from build123d import *

# Parameters (mm, degrees)
SKETCH1_R           = 3.95
BOSS_EXTRUDE1_DEPTH = 7.62
BOSS_EXTRUDE2_DEPTH = 7.62
BOSS_EXTRUDE3_DEPTH = 7.62
CUT_EXTRUDE1_DEPTH  = 7.62
SKETCH6_R           = 1.27
CUT_EXTRUDE2_DEPTH  = 4.9500048
SKETCH7_R           = 4.445
BOSS_EXTRUDE4_DEPTH = 1.27
FILLET1_R           = 2.54


with BuildPart() as part:
    # Sketch1 → Boss-Extrude1 (new body)
    with BuildSketch(Plane(origin=(0, 0, 0), x_dir=(0, 0, -1), z_dir=(1, 0, 0))):
        Circle(SKETCH1_R)
    extrude(amount=BOSS_EXTRUDE1_DEPTH)

    # Sketch2 → Boss-Extrude2 (add)
    with BuildSketch(Plane(origin=(7.62, 0, 0), x_dir=(0, 0, -1), z_dir=(1, 0, 0))):
        with BuildLine():
            Line((-3.95, 0), (-3.95, -10.16))
            Line((-3.95, -10.16), (3.95, -10.16))
            Line((3.95, -10.16), (3.95, 0))
            ThreePointArc((3.95, 0), (0, 3.95), (-3.95, 0))
        make_face()
    extrude(amount=BOSS_EXTRUDE2_DEPTH)

    # Sketch4 → Boss-Extrude3 (add)
    with BuildSketch(Plane(origin=(15.24, 0, 0), x_dir=(0, 0, -1), z_dir=(1, 0, 0))):
        with BuildLine():
            Line((-6.49, 0), (-6.49, -12.7))
            Line((-6.49, -12.7), (6.49, -12.7))
            Line((6.49, -12.7), (6.49, 0))
            ThreePointArc((6.49, 0), (0, 6.49), (-6.49, 0))
        make_face()
        with BuildLine():
            Line((-3.95, 0), (-3.95, -10.16))
            Line((-3.95, -10.16), (3.95, -10.16))
            Line((3.95, -10.16), (3.95, 0))
            ThreePointArc((3.95, 0), (0, 3.95), (-3.95, 0))
        make_face(mode=Mode.SUBTRACT)
    extrude(amount=-BOSS_EXTRUDE3_DEPTH)

    # Sketch5 → Cut-Extrude1 (cut)
    with BuildSketch(Plane(origin=(15.24, 0, 0), x_dir=(0, 0, -1), z_dir=(1, 0, 0))):
        with BuildLine():
            Line((-2.5399952, -2.54), (-2.5399952, -7.62))
            ThreePointArc((-2.5399952, -7.62), (4.8e-06, -10.16), (2.5400048, -7.62))
            Line((2.5400048, -7.62), (2.5400048, -2.54))
            ThreePointArc((2.5400048, -2.54), (4.8e-06, 0), (-2.5399952, -2.54))
        make_face()
    extrude(amount=-CUT_EXTRUDE1_DEPTH, mode=Mode.SUBTRACT)

    # Sketch6 → Cut-Extrude2 (cut, through all)
    with BuildSketch(Plane(origin=(0, 0, 2.5399952), x_dir=(-1, 0, 0), z_dir=(0, 0, -1))):
        with Locations((-11.290974186, -5.08)):
            Circle(SKETCH6_R)
    extrude(amount=-CUT_EXTRUDE2_DEPTH, mode=Mode.SUBTRACT)

    # Sketch7 → Boss-Extrude4 (add)
    with BuildSketch(Plane.ZY.offset(-7.62)):
        Circle(SKETCH7_R)
    extrude(amount=BOSS_EXTRUDE4_DEPTH)

    # Fillet1
    fillet1_edges = [part.edges().sort_by_distance(p)[0] for p in [
        (11.43, -12.7, -6.49),
        (11.43, -12.7, 6.49),
    ]]
    fillet(fillet1_edges, radius=FILLET1_R)


solid = part.part
Geometry check sheet. Reference: the model listing, model coordinates, mm. A direction names the side the tool comes from. Give positions to 0.01 mm unless a question says otherwise; leave off trailing zeros. Order: outer loops, then holes, each group sorted by start corner. A loop starts at its lowest first (then second) coordinate and runs counter-clockwise, first axis right, second up.
1) Tool access check on faces 5 (the cylindrical face through (11, 0, 0)), 6 (the cylindrical face through (10.12, -5.57, 4.49)), 7 (the flat face through (6.35, 4, -1)), 8 (the cylindrical face through (11.48, -10.16, 0.06)). Record the directions out of +Z, -Z, +X, -X, +Y, -Y that give a thin tool (end or side, any length) a straight path to the whole face; none if there is none.
Results are:
face 5: +X
face 6: +Z
face 7: -X
face 8: +X, -X
2) Material ranges on probe 1 along Z at (x, y) = (8.25, -5); probe 2 along Y at (x, z) = (13.25, 0); probe 3 along X at (y, z) = (4.75, 1), recorded low to high.
Results are:
probe 1: z = -6.49 to -2.54, 2.54 to 6.49
probe 2: y = -12.7 to -10.16, 0 to 6.49
probe 3: x = 7.62 to 15.24
3) Gauge pin test, flat ends, axial feed: pin 1 (1.5 mm diameter, centred on x = 2, z = 2, fed in from +Y); pin 2 (2 mm diameter, centred on y = -2.5, z = 0, fed in from +X); pin 3 (3 mm diameter, centred on x = 5.5, z = 4, fed in from -Y). Record the tip position at first contact, or that the pin passes through.
Results are:
pin 1: stops at y = 3.75
pin 2: stops at x = 7.62
pin 3: stops at y = -3.48
4) Cross-section at D-D (z = 3). Record the boundary of the cut face in (x, y) (3 decimals).
Results are:
outline: (0, -2.57) - (6.35, -2.57) - (6.35, -3.28) - (7.62, -3.28) - (7.62, -12.7) - (15.24, -12.7) - (15.24, 5.755) - (7.62, 5.755) - (7.62, 3.28) - (6.35, 3.28) - (6.35, 2.57) - (0, 2.57) - close; hole circle Ø2.54 at (11.291, -5.08)
5) Draft check along Z on faces 1 (the cylindrical face through (11.4, -12, 5.7)), 2 (the flat face through (7.62, -2, 0)), 3 (the cylindrical face through (11.4, -11.9, -5.8)), 4 (the flat face through (7.62, -5, 3)). Enter one of: released by +Z, released by -Z, zero draft, split by the parting line, or undercut.
Results are:
face 1: released by +Z
face 2: undercut
face 3: released by -Z
face 4: zero draft
6) Cross-section at A-A (z = 0). Record the boundary of the cut face in (x, y) (3 decimals).
Results are:
outline: (0, -3.95) - (6.35, -3.95) - (6.35, -4.445) - (7.62, -4.445) - (7.62, 0) - (15.24, 0) - (15.24, 6.49) - (7.62, 6.49) - (7.62, 4.445) - (6.35, 4.445) - (6.35, 3.95) - (0, 3.95) - close; (7.62, -12.7) - (15.24, -12.7) - (15.24, -10.16) - (7.62, -10.16) - close
7) Cross-section at C-C (y = -5.08). Record the boundary of the cut face in (x, z), then the cut area to 3 significant figures.
Results are:
outline: (7.62, -6.49) - (15.24, -6.49) - (15.24, -2.54) - (7.62, -2.54) - close; (7.62, 2.54) - (10.02, 2.54) - (10.02, 6.49) - (7.62, 6.49) - close; (12.56, 2.54) - (15.24, 2.54) - (15.24, 6.49) - (12.56, 6.49) - close
area: 50.2 mm2
8) Cross-section at B-B (x = 13.25). Record the boundary of the cut face in (y, z).
Results are:
outline: (-12.7, -3.95) arc R2.54 ccw to (-10.16, -6.49) - (0, -6.49) arc R6.49 ccw to (0, 6.49) - (-10.16, 6.49) arc R2.54 ccw to (-12.7, 3.95) - close; hole (-7.62, -2.54) - (-2.54, -2.54) arc R2.54 ccw to (-2.54, 2.54) - (-7.62, 2.54) arc R2.54 ccw to start
